Verification items for the finished model (mm, model axes). A direction names the side the tool comes from. Coordinates: 2 decimals unless noted, no trailing zeros. Write each loop counter-clockwise with the first axis right and the second up, starting at its lowest first coordinate (ties: lowest second). Pieces come first, ordered by that corner, then holes.
```python
from build123d import *

# Parameters (mm, degrees)
SKETCH1_W                     = 50.8
SKETCH1_H                     = 57.15
BOSS_EXTRUDE1_DEPTH           = 6.35
M5_CLEARANCE_HOLE1_D          = 5.5
M5_CLEARANCE_HOLE1_DEPTH      = 12.7
M5_CLEARANCE_HOLE1_TIP        = 1.652366702
TAP_DRILL_FOR_6_32_TAP1_D     = 2.7051
TAP_DRILL_FOR_6_32_TAP1_DEPTH = 12.7
TAP_DRILL_FOR_6_32_TAP1_TIP   = 0.81269403
TAP_DRILL_FOR_6_32_TAP2_D     = 2.7051
TAP_DRILL_FOR_6_32_TAP2_DEPTH = 12.7
TAP_DRILL_FOR_6_32_TAP2_TIP   = 0.81269403
FILLET1_R                     = 6.35
SKETCH8_R                     = 8
CUT_EXTRUDE1_DEPTH            = 6.35


with BuildPart() as part:
    # Sketch1 → Boss-Extrude1 (new body)
    with BuildSketch(Plane(origin=(0, 0, 0), x_dir=(1, 0, 0), z_dir=(0, 1, 0))):
        Rectangle(SKETCH1_W, SKETCH1_H)
    extrude(amount=BOSS_EXTRUDE1_DEPTH)

    # M5 Clearance Hole1
    with Locations(Plane(origin=(0, 6.35, 0), x_dir=(1, 0, 0), z_dir=(0, 1, 0))):
        with Locations((-16.167891819, 9.871960066), (-6.696960066, -12.992891819), (16.167891819, -3.521960066), (-6.696960066, 19.342891819), (6.696960066, 19.342891819), (16.167891819, 9.871960066), (-16.167891819, -3.521960066), (6.696960066, -12.992891819)):
            Hole(M5_CLEARANCE_HOLE1_D / 2, depth=M5_CLEARANCE_HOLE1_DEPTH)
            with Locations((0, 0, -(M5_CLEARANCE_HOLE1_DEPTH + M5_CLEARANCE_HOLE1_TIP / 2))):  # 118° drill point
                Cone(0, M5_CLEARANCE_HOLE1_D / 2, M5_CLEARANCE_HOLE1_TIP, mode=Mode.SUBTRACT)

    # Tap Drill for #6-32 Tap1
    with Locations(Plane.XY.offset(28.575)):
        with Locations((-15.875, 3.175), (15.875, 3.175)):
            Hole(TAP_DRILL_FOR_6_32_TAP1_D / 2, depth=TAP_DRILL_FOR_6_32_TAP1_DEPTH)
            with Locations((0, 0, -(TAP_DRILL_FOR_6_32_TAP1_DEPTH + TAP_DRILL_FOR_6_32_TAP1_TIP / 2))):  # 118° drill point
                Cone(0, TAP_DRILL_FOR_6_32_TAP1_D / 2, TAP_DRILL_FOR_6_32_TAP1_TIP, mode=Mode.SUBTRACT)

    # Tap Drill for #6-32 Tap2
    with Locations(Plane(origin=(25.4, 0, 0), x_dir=(0, 0, -1), z_dir=(1, 0, 0))):
        with Locations((-9.525, 3.175), (19.05, 3.175)):
            Hole(TAP_DRILL_FOR_6_32_TAP2_D / 2, depth=TAP_DRILL_FOR_6_32_TAP2_DEPTH)
            with Locations((0, 0, -(TAP_DRILL_FOR_6_32_TAP2_DEPTH + TAP_DRILL_FOR_6_32_TAP2_TIP / 2))):  # 118° drill point
                Cone(0, TAP_DRILL_FOR_6_32_TAP2_D / 2, TAP_DRILL_FOR_6_32_TAP2_TIP, mode=Mode.SUBTRACT)

    # Fillet1
    fillet1_edges = [part.edges().sort_by_distance(p)[0] for p in [
        (-25.4, 3.175, -28.575),
    ]]
    fillet(fillet1_edges, radius=FILLET1_R)

    # Sketch8 → Cut-Extrude1 (cut)
    with BuildSketch(Plane(origin=(0, 6.35, 0), x_dir=(1, 0, 0), z_dir=(0, 1, 0))):
        with Locations(Location((0, 3.175, 0), (0, 0, 270))):
            Circle(SKETCH8_R)
    extrude(amount=-CUT_EXTRUDE1_DEPTH, mode=Mode.SUBTRACT)


solid = part.part
```
1. Tool access check on faces 1 (the cylindrical face through (-14.524, 3.234, 22.136)), 2 (the cylindrical face through (18.96, 3.58, -17.76)), 3 (the cylindrical face through (-4.515, 3.131, -17.67)). Record the directions out of +Z, -Z, +X, -X, +Y, -Y that give a thin tool (end or side, any length) a straight path to the whole face; none if there is none.
2. Sectioned sample at C-C, the plane y = 2.5. Give the number of separate pieces and of enclosed holes in the cut face, and give its area (3 significant figures).
3. Material ranges on L1, parallel to Z at x = 7, y = 6.25 (3 decimals); L2, parallel to X at y = 3.75, z = 16.5; L3, parallel to X at y = 2, z = 13.5, recorded low to high.
4. Sectioned sample at B-B, the plane z = -6. Record the boundary of the cut face in (x, y), and give its area (3 significant figures).
5. Draft check along Z on faces 4 (the conical face through (-15.651, 3.246, 15.203)), 5 (the flat face through (0, 6.35, 6)), 6 (the cylindrical face through (-7.81, 3.22, -4.91)), 7 (the cylindrical face through (-23.589, 3.219, -26.665)). Enter one of: pulls with the +Z half, pulls with the -Z half, needs draft (parallel to the pull), parting line crosses it, or undercut.
6. Sectioned sample at A-A, the plane x = 0. Record the boundary of the cut face in (y, z) (3 decimals).
7. Gauge pin test, flat end, axial feed: P1, Ø10, axis at x = 10.5, z = 7.5, coming from the -Y side. Record the tip position at first contact, or that the pin passes through.
Outcome:
1. face 1: +Z
1. face 2: +X
1. face 3: +Y, -Y
2. separate pieces: 1
2. enclosed holes: 9
2. area: 2,380 mm2
3. L1: z = -28.575 to -22.076, -16.61 to -7.048, 0.698 to 10.26, 15.726 to 28.575
3. L2: x = -25.4 to -17.1, -14.65 to 14.65, 17.1 to 25.4
3. L3: x = -25.4 to -9.4, -3.99 to 3.99, 9.4 to 25.4
4. outline: (-25.4, 0) - (-7.48, 0) - (-7.48, 6.35) - (-25.4, 6.35) - close; (7.48, 0) - (25.4, 0) - (25.4, 6.35) - (7.48, 6.35) - close
4. area: 228 mm2
5. face 4: pulls with the +Z half
5. face 5: needs draft
5. face 6: undercut
5. face 7: pulls with the -Z half
6. outline: (0, -28.575) - (6.35, -28.575) - (6.35, -11.175) - (0, -11.175) - close; (0, 4.825) - (6.35, 4.825) - (6.35, 28.575) - (0, 28.575) - close
7. P1: stops at y = 0
